```python
from build123d import *

# Parameters (mm, degrees)
SKETCH2_R           = 1.75
BOSS_EXTRUDE3_DEPTH = 5


with BuildPart() as part:
    # Sketch2 → Boss-Extrude3 (new body)
    with BuildSketch(Plane(origin=(0, 0, 0), x_dir=(1, 0, 0), z_dir=(0, 1, 0))):
        Polygon((-268, -48.75), (-268, -56.75), (-254, -56.75), (-254, -48.75), (-261, -44.75), align=None)
        with Locations((-261, -50)):
            Circle(SKETCH2_R, mode=Mode.SUBTRACT)
    extrude(amount=BOSS_EXTRUDE3_DEPTH)


solid = part.part
```
Design review of the part built by this model. Coordinates are the model's own, in mm. Give positions to 0.01 mm unless a question says otherwise; leave off trailing zeros. Loops run counter-clockwise (first coordinate to the right, second up) from the corner with the lowest first, then second, coordinate; pieces in that order, holes last. Notation, with made-up numbers: M -1.75,14 L 7.25,14 A17 ccw 7.25,20 Z; hole C 31,55 d9. An arc over 180 degrees is marked long. Return JSON: item names as keys, results as strings. Group by question number.
Item 1: Insertion check: pin 1 Ø5 at (x, z) = (-265, 47) entering from +Y. The pin has a flat end and moves straight along its axis. Give the tip position at first contact, or say it passes through.
Item 2: We need section A-A (z = 50). Give the boundary of the cut face in (x, y), and give its area (3 significant figures).
Item 3: For probe 1 along X at (y, z) = (3.35, 50); probe 2 along X at (y, z) = (0.55, 45.75); probe 3 along Z at (x, y) = (-262.5, 4), list the stretches that pass through material, from the lowest coordinate up.
Item 4: We need section B-B (y = 4.75). Give the boundary of the cut face in (x, z).
Item 5: We need section D-D (z = 47.75). Give the boundary of the cut face in (x, y).
Item 6: Mouldability with a two-part tool opening along Z and no side actions: class faces 1 (the flat face through (-264.45, 2.46, 46.72)), 2 (the flat face through (-261, 2, 56.75)), 3 (the flat face through (-268, 2, 53)), 4 (the cylindrical face through (-262.39, 2.46, 51.06)) as released by +Z, released by -Z, zero draft, split by the parting line, or undercut.
Item 7: We need section C-C (x = -259.75). Give the boundary of the cut face in (y, z).
Output:
{
 "1": {"pin 1": "stops at y = 5"},
 "2": {"outline": "M -268,0 L -262.75,0 L -262.75,5 L -268,5 Z; M -259.25,0 L -254,0 L -254,5 L -259.25,5 Z", "area": "52.5 mm^2"},
 "3": {"probe 1": "x = -268 to -262.75, -259.25 to -254", "probe 2": "x = -262.75 to -259.25", "probe 3": "z = 45.61 to 49.1, 50.9 to 56.75"},
 "4": {"outline": "M -268,48.75 L -261,44.75 L -254,48.75 L -254,56.75 L -268,56.75 Z; hole C -261,50 d3.5"},
 "5": {"outline": "M -266.25,0 L -255.75,0 L -255.75,5 L -266.25,5 Z"},
 "6": {"face 1": "released by -Z", "face 2": "released by +Z", "face 3": "zero draft", "face 4": "undercut"},
 "7": {"outline": "M 0,45.46 L 5,45.46 L 5,48.78 L 0,48.78 Z; M 0,51.22 L 5,51.22 L 5,56.75 L 0,56.75 Z"}
}
